The model under review builds one solid part; all positions refer to its coordinate system, in mm. A direction names the side the tool comes from. Round coordinates to 2 decimals unless told otherwise and drop trailing zeros. Order: outer loops, then holes, each group sorted by start corner. A loop starts at its lowest first (then second) coordinate and runs counter-clockwise, first axis right, second up. Notation, with made-up numbers: M 73,6.25 L 105,6.25 A25 ccw 105,18.25 Z; hole C 53,46 d1. An arc over 180 degrees is marked long. Use a Markdown table: item, result. Add a question column.
1. For faces 1 (the flat face through (136.471, -159.017, 3.131)), 2 (the flat face through (3, 2, 0)), 3 (the flat face through (-136.471, 159.017, 3.131)), list the 3-axis set-ups (+Z, -Z, +X, -X, +Y, -Y) from which the entire face can be reached by the end or side of a thin tool; tool diameter is ignored.
2. Consider section C-C on x = 162.5. State the section outline as (y, z) points, then the cut area to 3 significant figures.
3. The part is to be moulded in two halves that separate along X. For faces 4 (the flat face through (3, 2, 6.35)), 5 (the flat face through (-133.404, -158.483, 3.131)), say which applies: +X half, -X half, draft (parallel to the pull), parting line (faces both ways), or undercut.
4. Insertion check: P1, Ø3, axis at x = -5, z = 2, coming from the +Y side. The pin has a flat end and moves straight along its axis. Give the tip position at first contact, or say it passes through.
5. Consider section A-A on z = 4.75. State the section outline as (x, y) points (3 decimals).
6. To check wall thickness, follow probe 1 along Y at (x, z) = (11, 5.5); probe 2 along Y at (x, z) = (-95, 3.25). State the ranges of each line that lie inside material, in increasing order.
7. Consider section B-B on x = -43. State the section outline as (y, z) points.
from build123d import *

# Parameters (mm, degrees)
SKETCH2_W           = 50.8
SKETCH2_H           = 279.4
BOSS_EXTRUDE2_DEPTH = 6.35


with BuildPart() as part:
    # Sketch2 → Boss-Extrude2 (new body)
    with BuildSketch(Plane.XY):
        Polygon((-25.4, -139.7), (-244.475, -177.8), (-244.475, 177.8), (-25.4, 139.7), align=None)
        Rectangle(SKETCH2_W, SKETCH2_H)
        Polygon((25.4, -139.7), (25.4, 139.7), (244.475, 177.8), (244.475, -177.8), align=None)
    extrude(amount=BOSS_EXTRUDE2_DEPTH)


solid = part.part
Answer block:
| question | item | result |
|---|---|---|
| 1 | face 1 | +Z, -Z, -Y |
| 1 | face 2 | -Z, +X, -X, +Y, -Y |
| 1 | face 3 | +Z, -Z, +Y |
| 2 | outline | M -163.54,0 L 163.54,0 L 163.54,6.35 L -163.54,6.35 Z |
| 2 | area | 2,080 mm^2 |
| 3 | face 4 | draft |
| 3 | face 5 | undercut |
| 4 | P1 | y = 139.7 |
| 5 | outline | M -244.475,-177.8 L -25.4,-139.7 L 25.4,-139.7 L 244.475,-177.8 L 244.475,177.8 L 25.4,139.7 L -25.4,139.7 L -244.475,177.8 Z |
| 6 | probe 1 | -139.7 to 139.7 |
| 6 | probe 2 | -151.8 to 151.8 |
| 7 | outline | M -142.76,0 L 142.76,0 L 142.76,6.35 L -142.76,6.35 Z |
